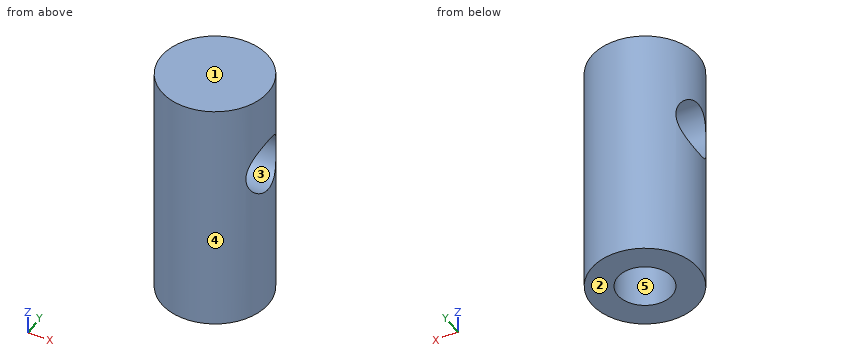
```python
from build123d import *

# Parameters (mm, degrees)
F0_R     = 7.85
F1_DEPTH = 35
F2_R     = 4
F3_DEPTH = 12.5
F4_R     = 4
F5_DEPTH = 18


with BuildPart() as f1:
    # F0 (on Top) → F1 (new body)
    with BuildSketch(Plane.XY):
        Circle(F0_R)
    extrude(amount=F1_DEPTH)

    # F2 (on Right) → F3 (cut, symmetric)
    with BuildSketch(Plane.YZ):
        with Locations((0, 23)):
            Circle(F2_R)
    extrude(amount=F3_DEPTH, both=True, mode=Mode.SUBTRACT)

    # F4 (on face) → F5 (cut)
    with BuildSketch(Plane(origin=(0, 0, 0), x_dir=(1, 0, 0), z_dir=(0, 0, -1))):
        Circle(F4_R)
    extrude(amount=-F5_DEPTH, mode=Mode.SUBTRACT)


solid = f1.part
```
Can you work these out from the model? Positions are in its coordinate system, mm. Face numbers are marked on the shaded views. A direction names the side the tool comes from. Coordinates: 2 decimals unless noted, no trailing zeros. Write each loop counter-clockwise with the first axis right and the second up, starting at its lowest first coordinate (ties: lowest second). Pieces come first, ordered by that corner, then holes. Notation, with made-up numbers: M 54.5,34.25 L 106.5,34.25 A16 ccw 106.5,43.25 Z; hole C 67,-8 d3. An arc over 180 degrees is marked long. Write item = value, one per line. Start each with the question number.
Q1. If we section it at D-D, the plane z = 3: Write out the boundary of the cut face in (x, y).
Q2. If we section it at A-A, the plane x = 0: Write out the boundary of the cut face in (y, z), then the cut area to 3 significant figures.
Q3. On a 3-axis mill with a long thin cutter (end or side, diameter ignored), from which of +Z, -Z, +X, -X, +Y, -Y can I reach the whole of each face in a straight line? I mean the marked faces 4 and 5. Say none if no direction works.
Q4. If we section it at C-C, the plane x = 7.25: Write out the boundary of the cut face in (y, z).
Q5. Thinking about a two-plate mould opening in Z: for the marked faces 1, 2 and 3, which applies, released by +Z, released by -Z, zero draft, split by the parting line, or undercut?
Q6. If I drill on L1, parallel to Y at x = 0, z = 11.25; L2, parallel to Z at x = -1.5, y = 0, over which ranges is the centre line in solid material (lowest first)? Write a range as [from, to].
Q7. If we section it at B-B, the plane y = 0: Write out the boundary of the cut face in (x, z), then the cut area to 3 significant figures.
Q8. I'm going to push flat-ended pins straight in: pin 1 (1.5 mm diameter, centred on x = -6, z = 6.5, fed in from -Y); pin 2 (1 mm diameter, centred on y = -2, z = 4, fed in from +X); pin 3 (2.5 mm diameter, centred on x = 1, y = 0, fed in from -Z). Where does each tip first touch, or does it pass through?
Check sheet entries:
q1.outline = C 0,0 d15.7; hole C 0,0 d8
q2.outline = M -7.85,0 L -4,0 L -4,18 L 4,18 L 4,0 L 7.85,0 L 7.85,35 L -7.85,35 Z; hole C 0,23 d8
q2.area = 355 mm²
q3.face_4 = +Z, -Z
q3.face_5 = -Z
q4.outline = M -3.01,0 L 3.01,0 L 3.01,20.37 A4 cw -3.01,20.37 Z; M -3.01,25.63 A4 cw 3.01,25.63 L 3.01,35 L -3.01,35 Z
q5.face_1 = released by +Z
q5.face_2 = released by -Z
q5.face_3 = undercut
q6.L1 = [-7.85, -4], [4, 7.85]
q6.L2 = [18, 19], [27, 35]
q7.outline = M -7.85,0 L -4,0 L -4,18 L 4,18 L 4,0 L 7.85,0 L 7.85,19 L -7.85,19 Z; M -7.85,27 L 7.85,27 L 7.85,35 L -7.85,35 Z
q7.area = 280 mm²
q8.pin_1 = -5.84
q8.pin_2 = 7.71
q8.pin_3 = 18
